Part model, mm, in its own coordinate system. Face numbers are marked on the shaded views. A direction names the side the tool comes from. Give positions to 0.01 mm unless a question says otherwise; leave off trailing zeros. Write each loop counter-clockwise with the first axis right and the second up, starting at its lowest first coordinate (ties: lowest second). Pieces come first, ordered by that corner, then holes.
```python
from build123d import *

# Parameters (mm, degrees)
CROQUIS1_R              = 18.4
SALIENTE_EXTRUIR1_DEPTH = 24.3
CROQUIS2_R              = 3
CROQUIS2_R_2            = 1.25
CORTAR_EXTRUIR1_DEPTH   = 5
CORTAR_EXTRUIR2_START   = -5
CROQUIS3_R              = 1.25
CROQUIS3_R_2            = 5
CORTAR_EXTRUIR2_DEPTH   = 5
CORTAR_EXTRUIR3_START   = -5
CROQUIS6_R              = 18.4
CORTAR_EXTRUIR3_DEPTH   = 5
CROQUIS7_R              = 6
CORTAR_EXTRUIR4_DEPTH   = 1


with BuildPart() as part:
    # Croquis1 → Saliente-Extruir1 (new body)
    with BuildSketch(Plane.XY):
        Circle(CROQUIS1_R)
    extrude(amount=SALIENTE_EXTRUIR1_DEPTH)

    # Croquis2 → Cortar-Extruir1 (cut)
    with BuildSketch(Plane.XY.offset(24.3)):
        Circle(CROQUIS2_R)
        with Locations((0, 9.5)):
            Circle(CROQUIS2_R_2)
        with Locations((9.5, 0)):
            Circle(CROQUIS2_R_2)
        with Locations((0, -9.5)):
            Circle(CROQUIS2_R_2)
        with Locations((-9.5, 0)):
            Circle(CROQUIS2_R_2)
    extrude(amount=-CORTAR_EXTRUIR1_DEPTH, mode=Mode.SUBTRACT)

    # Croquis3 → Cortar-Extruir2 (cut)
    with BuildSketch(Plane(origin=(0, 0, 0), x_dir=(-1, 0, 0), z_dir=(0, 0, -1)).offset(CORTAR_EXTRUIR2_START)):
        with Locations(Location((-9.5, 0, 0), (0, 0, 180))):
            Circle(CROQUIS3_R)
        with Locations(Location((0, 9.5, 0), (0, 0, 180))):
            Circle(CROQUIS3_R)
        with Locations(Location((9.5, 0, 0), (0, 0, 180))):
            Circle(CROQUIS3_R)
        with Locations(Location((0, -9.5, 0), (0, 0, 180))):
            Circle(CROQUIS3_R)
        Circle(CROQUIS3_R_2)
    extrude(amount=CORTAR_EXTRUIR2_DEPTH, mode=Mode.SUBTRACT)

    # Croquis6 → Cortar-Extruir3 (cut)
    with BuildSketch(Plane.XY.offset(24.3).offset(CORTAR_EXTRUIR3_START)):
        Circle(CROQUIS6_R)
    extrude(amount=CORTAR_EXTRUIR3_DEPTH, mode=Mode.SUBTRACT)

    # Croquis7 → Cortar-Extruir4 (cut)
    with BuildSketch(Plane.XY.offset(19.3)):
        Circle(CROQUIS7_R)
    extrude(amount=-CORTAR_EXTRUIR4_DEPTH, mode=Mode.SUBTRACT)


solid = part.part
```
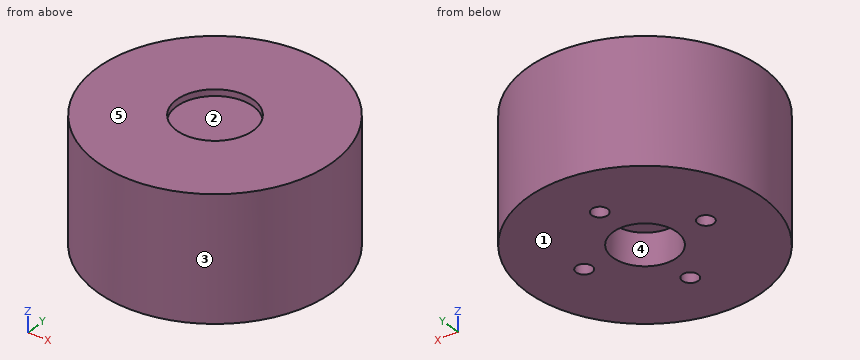
1) Saw through at D-D, the plane x = 9.5. Write the cut outline in (y, z), then the cut area to 3 significant figures.
Answers follow:
outline: (-15.76, 0) - (-1.25, 0) - (-1.25, 5) - (1.25, 5) - (1.25, 0) - (15.76, 0) - (15.76, 19.3) - (-15.76, 19.3) - close
area: 596 mm2
2) Saw through at C-C, the plane z = 16.25. Write the cut outline in (x, y).
Answers follow:
outline: circle Ø36.8 at (0, 0)
3) Wall check: L1, parallel to Y at x = 0, z = 2.75; L2, parallel to Y at x = 8.5, z = 1.5; L3, parallel to Z at x = -3.5, y = 0. Give the ranges that are in metal, low to high.
Answers follow:
L1: y = -18.4 to -10.75, -8.25 to -5, 5 to 8.25, 10.75 to 18.4
L2: y = -16.32 to -0.75, 0.75 to 16.32
L3: z = 5 to 18.3
4) 3-axis set-ups, long thin cutter, end or side, ignore diameter. For the marked faces 1 and 2: which of +Z, -Z, +X, -X, +Y, -Y reach the whole face in a straight line?
Answers follow:
face 1: -Z, +X, -X, +Y, -Y
face 2: +Z
5) Saw through at B-B, the plane y = -5.5. Write the cut outline in (x, z).
Answers follow:
outline: (-17.56, 0) - (17.56, 0) - (17.56, 19.3) - (2.4, 19.3) - (2.4, 18.3) - (-2.4, 18.3) - (-2.4, 19.3) - (-17.56, 19.3) - close
6) Saw through at A-A, the plane x = 0. Write the cut outline in (y, z), then the cut area to 3 significant figures.
Answers follow:
outline: (-18.4, 0) - (-10.75, 0) - (-10.75, 5) - (-8.25, 5) - (-8.25, 0) - (-5, 0) - (-5, 5) - (5, 5) - (5, 0) - (8.25, 0) - (8.25, 5) - (10.75, 5) - (10.75, 0) - (18.4, 0) - (18.4, 19.3) - (6, 19.3) - (6, 18.3) - (-6, 18.3) - (-6, 19.3) - (-18.4, 19.3) - close
area: 623 mm2
7) Pin check, flat tips, straight feed: pin 1 Ø11 at (x, y) = (0, 0) entering from +Z; pin 2 Ø5 at (y, z) = (-9.5, 16.5) entering from +X; pin 3 Ø3 at (x, y) = (-1, 2.5) entering from -Z. Stop position of each tip, or through.
Answers follow:
pin 1: stops at z = 18.3
pin 2: stops at x = 17.02
pin 3: stops at z = 5
8) Two-plate mould, pull along X, no slides. Class the marked faces 3, 4 and 5: +X half, -X half, draft (parallel to the pull), parting line (faces both ways), or undercut.
Answers follow:
face 3: parting line
face 4: undercut
face 5: draft
